Model file for the job. Use its own axes, mm. Round coordinates to 2 decimals unless told otherwise and drop trailing zeros. Loops run counter-clockwise (first coordinate to the right, second up) from the corner with the lowest first, then second, coordinate; pieces in that order, holes last. Notation, with made-up numbers: M 13,88.5 L 31,88.5 A18 cw 31,114.5 Z; hole C 80,-37.75 d9. An arc over 180 degrees is marked long. Answer in a Markdown table with one row per item.
from build123d import *

# Parameters (mm, degrees)
F0_W           = 170
F0_H           = 35
F1_DEPTH       = 10
F2_D           = 6
F2_DEPTH       = 40
F2_TIP         = 1.8025818571
F3_D           = 8.8
F3_DEPTH       = 40
F3_CSINK_D     = 17.92
F3_CSINK_ANGLE = 90
F3_TIP         = 2.6437867237
F5_D           = 5.25
F5_DEPTH       = 40
F5_TIP         = 1.5772591249


with BuildPart() as f1:
    # F0 (on Front) → F1 (new body)
    with BuildSketch(Plane.XZ):
        Polygon((37, 35), (37, 53), (-37, 53), (-37, -53), (37, -53), (37, -35), (37, 0), align=None)
        with Locations((122, -17.5)):
            Rectangle(F0_W, F0_H)
        with Locations((122, 17.5)):
            Rectangle(F0_W, F0_H)
    extrude(amount=F1_DEPTH)

    # F2
    with Locations(Plane(origin=(0, 0, 0), x_dir=(1, 0, 0), z_dir=(0, 1, 0))):
        with Locations((-29, 0), (29, 0)):
            Hole(F2_D / 2, depth=F2_DEPTH)
            with Locations((0, 0, -(F2_DEPTH + F2_TIP / 2))):  # 118° drill point
                Cone(0, F2_D / 2, F2_TIP, mode=Mode.SUBTRACT)

    # F3
    with Locations(Plane(origin=(0, 0, 0), x_dir=(1, 0, 0), z_dir=(0, 1, 0))):
        with Locations((29, 30), (-29, 30), (29, -30), (-29, -30)):
            CounterSinkHole(F3_D / 2, F3_CSINK_D / 2, depth=F3_DEPTH, counter_sink_angle=F3_CSINK_ANGLE)
            with Locations((0, 0, -(F3_DEPTH + F3_TIP / 2))):  # 118° drill point
                Cone(0, F3_D / 2, F3_TIP, mode=Mode.SUBTRACT)

    # F5
    with Locations(Plane(origin=(0, 0, 0), x_dir=(1, 0, 0), z_dir=(0, 1, 0))):
        with Locations((0, 30), (0, -30), (200, 30), (200, -30)):
            Hole(F5_D / 2, depth=F5_DEPTH)
            with Locations((0, 0, -(F5_DEPTH + F5_TIP / 2))):  # 118° drill point
                Cone(0, F5_D / 2, F5_TIP, mode=Mode.SUBTRACT)


solid = f1.part
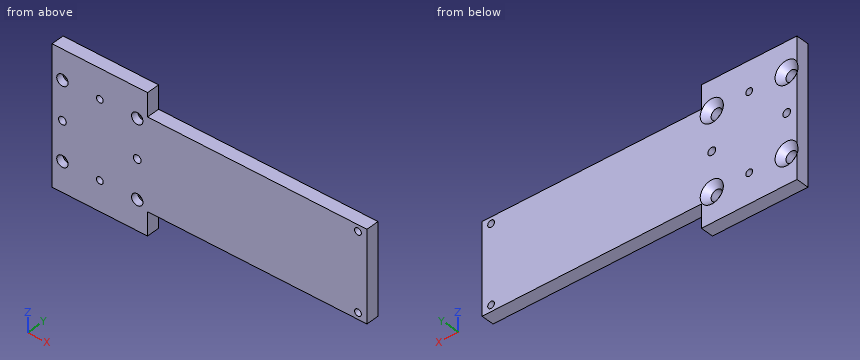
1. Saw through at A-A (x = 200). Write the cut outline in (y, z) (3 decimals), and give its area (3 significant figures).
Verdict:
| item | result |
|---|---|
| outline | M -10,-35 L 0,-35 L 0,-32.625 L -10,-32.625 Z; M -10,-27.375 L 0,-27.375 L 0,27.375 L -10,27.375 Z; M -10,32.625 L 0,32.625 L 0,35 L -10,35 Z |
| area | 595 mm² |
2. Saw through at C-C (x = -29). Write the cut outline in (y, z).
Verdict:
| item | result |
|---|---|
| outline | M -10,-53 L 0,-53 L 0,-38.96 L -4.56,-34.4 L -10,-34.4 Z; M -10,-25.6 L -4.56,-25.6 L 0,-21.04 L 0,-3 L -10,-3 Z; M -10,3 L 0,3 L 0,21.04 L -4.56,25.6 L -10,25.6 Z; M -10,34.4 L -4.56,34.4 L 0,38.96 L 0,53 L -10,53 Z |
3. Pin check, flat tips, straight feed: pin 1 (14 mm diameter, centred on x = 29, z = 30, fed in from +Y); pin 2 (8.5 mm diameter, centred on x = 0, z = 30, fed in from +Y); pin 3 (5 mm diameter, centred on x = 75, y = -5.5, fed in from +Z); pin 4 (10 mm diameter, centred on x = -29, z = 30, fed in from +Y). Stop position of each tip, or through.
Verdict:
| item | result |
|---|---|
| pin 1 | stops at y = -1.96 |
| pin 2 | stops at y = 0 |
| pin 3 | stops at z = 35 |
| pin 4 | stops at y = -3.96 |
4. Wall check: probe 1 along Z at (x, y) = (-29, -6.5); probe 2 along Z at (x, y) = (200, -2.5) (3 decimals); probe 3 along X at (y, z) = (-6.3, -30) (3 decimals). Give the ranges that are in metal, low to high.
Verdict:
| item | result |
|---|---|
| probe 1 | z = -53 to -34.4, -25.6 to -3, 3 to 25.6, 34.4 to 53 |
| probe 2 | z = -35 to -32.625, -27.375 to 27.375, 32.625 to 35 |
| probe 3 | x = -37 to -33.4, -24.6 to -2.625, 2.625 to 24.6, 33.4 to 197.375, 202.625 to 207 |
5. Saw through at D-D (z = -30). Write the cut outline in (x, y) (3 decimals).
Verdict:
| item | result |
|---|---|
| outline | M -37,-10 L -33.4,-10 L -33.4,-4.56 L -37,-0.96 Z; M -24.6,-10 L -2.625,-10 L -2.625,0 L -20.04,0 L -24.6,-4.56 Z; M 2.625,-10 L 24.6,-10 L 24.6,-4.56 L 20.04,0 L 2.625,0 Z; M 33.4,-10 L 197.375,-10 L 197.375,0 L 37.96,0 L 33.4,-4.56 Z; M 202.625,-10 L 207,-10 L 207,0 L 202.625,0 Z |
6. Saw through at B-B (y = -3). State how many separate pieces and enclosed holes the cut face has, and give its area (3 significant figures).
Verdict:
| item | result |
|---|---|
| separate pieces | 1 |
| enclosed holes | 10 |
| area | 19,200 mm² |
